Source: CAD feature listing. Evaluate the final solid. Frame: model axes, mm. Face numbers are marked on the shaded views. A direction names the side the tool comes from. Round coordinates to 2 decimals unless told otherwise and drop trailing zeros. Loops run counter-clockwise (first coordinate to the right, second up) from the corner with the lowest first, then second, coordinate; pieces in that order, holes last. Notation, with made-up numbers: M 27.25,44.25 L 47.25,44.25 A21 ccw 47.25,61.25 Z; hole C 26.25,53.5 d4. An arc over 180 degrees is marked long. One line per item, written item: value.
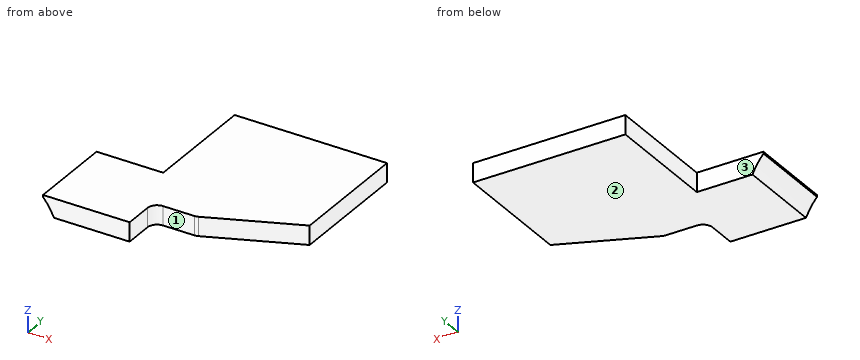
from build123d import *

# Parameters (mm, degrees)
SKETCH1_W           = 80
SKETCH1_H           = 65
BOSS_EXTRUDE1_DEPTH = 10
SKETCH3_W           = 80
SKETCH3_H           = 10
BOSS_EXTRUDE2_DEPTH = 40
SKETCH4_W           = 10
SKETCH4_H           = 45
BOSS_EXTRUDE3_DEPTH = 35
SKETCH5_R           = 36.5
CUT_EXTRUDE2_DEPTH  = 97.566039579
CUT_EXTRUDE3_DEPTH  = 105.791459576


with BuildPart() as part:
    # Sketch1 → Boss-Extrude1 (new body)
    with BuildSketch(Plane.XY):
        Rectangle(SKETCH1_W, SKETCH1_H)
    extrude(amount=BOSS_EXTRUDE1_DEPTH)

    # Sketch3 → Boss-Extrude2 (add)
    with BuildSketch(Plane.XZ.offset(32.5)):
        with Locations((0, 5)):
            Rectangle(SKETCH3_W, SKETCH3_H)
    extrude(amount=BOSS_EXTRUDE2_DEPTH)

    # Sketch4 → Boss-Extrude3 (add)
    with BuildSketch(Plane.ZY.offset(40)):
        with Locations((5, -50)):
            Rectangle(SKETCH4_W, SKETCH4_H)
    extrude(amount=BOSS_EXTRUDE3_DEPTH)

    # Sketch5 → Cut-Extrude2 (cut, through all)
    with BuildSketch(Plane(origin=(0, -27.5, 0), x_dir=(1, 0, 0), z_dir=(0, 1, 0))):
        with Locations((-102.5, 15)):
            Circle(SKETCH5_R)
    extrude(amount=-CUT_EXTRUDE2_DEPTH, mode=Mode.SUBTRACT)

    # Sketch6 → Cut-Extrude3 (cut, through all)
    with BuildSketch(Plane.XY.offset(10)):
        with BuildLine():
            Line((-29.5, -72.5), (40, -72.5))
            Line((40, -72.5), (40, -32.5))
            Line((40, -32.5), (-6.061816969, -52.100773178))
            ThreePointArc((-6.061816969, -52.100773178), (-7.020559729, -52.399176762), (-8.019592789, -52.5))
            Line((-8.019592789, -52.5), (-24.5, -52.5))
            ThreePointArc((-24.5, -52.5), (-28.035533906, -53.964466094), (-29.5, -57.5))
            Line((-29.5, -57.5), (-29.5, -72.5))
        make_face()
    extrude(amount=-CUT_EXTRUDE3_DEPTH, mode=Mode.SUBTRACT)


solid = part.part
1. Pin query (flat end, axial travel): pin 1 (5 mm diameter, centred on y = -5, z = 7, fed in from -X); pin 2 (6 mm diameter, centred on x = -43.5, z = 7, fed in from +Y). Return the tip coordinate at first contact, or that it passes through.
Report:
pin 1: stops at x = -40
pin 2: stops at y = -27.5
2. Reachability of the marked faces 1, 2 and 3 from +Z, -Z, +X, -X, +Y, -Y: full face, straight path, thin tool, end or side. Return the list, or none.
Report:
face 1: +Z, -Z, +X, -Y
face 2: -Z, +X, -X, +Y, -Y
face 3: +Z, -Z, -X, +Y
3. Section query A-A (z = 6.75). Return the cut outline in (x, y), and give its area (3 significant figures).
Report:
outline: M -73.19,-72.5 L -29.5,-72.5 L -29.5,-57.5 A5 cw -24.5,-52.5 L -8.02,-52.5 A5 ccw -6.06,-52.1 L 40,-32.5 L 40,32.5 L -40,32.5 L -40,-27.5 L -73.19,-27.5 Z
area: 8,040 mm2
4. Ray query, line 1 (X direction, y = 5.5, z = 7.5); line 2 (Y direction, x = -25, z = 1); line 3 (X direction, y = -58, z = 9.5). Return the intervals inside material, ascending. Write a range as [from, to].
Report:
line 1: x = [-40, 40]
line 2: y = [-52.53, 32.5]
line 3: x = [-75, -29.5]
5. Section query C-C (x = -67.5). Return the cut outline in (y, z), and give its area (3 significant figures).
Report:
outline: M -72.5,0 L -27.5,0 L -27.5,10 L -72.5,10 Z
area: 450 mm2
6. Section query B-B (y = -60.5). Return the cut outline in (x, z), and give its area (3 significant figures).
Report:
outline: M -75,9 A36.5 cw -69.22,0 L -29.5,0 L -29.5,10 L -75,10 Z
area: 426 mm2
7. Section query D-D (y = -34). Return the cut outline in (x, z) (3 decimals), and give its area (3 significant figures).
Report:
outline: M -75,9 A36.5 cw -69.225,0 L 36.475,0 L 36.475,10 L -75,10 Z
area: 1,090 mm2
